from build123d import *

# Parameters (mm, degrees)
F1_W         = 18.1
F1_H         = 18.1
F2_DEPTH     = 5
F3_W         = 16.1
F3_H         = 16.1
F4_DEPTH     = 4
F5_ANGLE     = 45
F7_DEPTH     = 5
F9_DEPTH     = 8
F10_T1_DEPTH = 17.995241473
F11_T1_DEPTH = 15.801577482
F11_T3_DEPTH = 15.801577482
F11_T6_ANGLE = 128.9448568851
F11_T8_ANGLE = 128.9448568851


# Not quite as in the source:
# - a fillet or chamfer that OpenCascade refuses, or shapes differently, is made with other operations: its cross-section is extruded or revolved along the edge and cut away or added


with BuildPart() as f2:
    # F1 (on Top) → F2 (new body)
    with BuildSketch(Plane.XY):
        Rectangle(F1_W, F1_H)
    extrude(amount=F2_DEPTH)

    # F3 (on Top) → F4 (cut)
    with BuildSketch(Plane.XY):
        Rectangle(F3_W, F3_H)
    extrude(amount=F4_DEPTH, mode=Mode.SUBTRACT)


with BuildPart() as f2_1:
    # F5: moved
    add(f2.part.rotate(Axis((0, 0, 23.8891355693), (0, 0, 1)), F5_ANGLE))

    # F6 (on face) → F7 (join)
    with BuildSketch(Plane.XY.offset(5)):
        Polygon((12.7986327395, 0), (6.3993163697, -6.3993163697), (16.6505072266, 0), (6.3993163697, 6.3993163697), align=None)
    extrude(amount=-F7_DEPTH)

    # F8 (on face) → F9 (join)
    with BuildSketch(Plane(origin=(0, 0, 0), x_dir=(1, 0, 0), z_dir=(0, 0, -1))):
        Polygon((16.6505072266, 0), (6.3993163697, 6.3993163697), (6.3993163697, 4.9851028074), (11.3844191771, 0), (6.3993163697, -4.9851028074), (6.3993163697, -6.3993163697), align=None)
    extrude(amount=F9_DEPTH)

    # F10: fillet of radius 5 on 2 edges, made by hand

    # F10_s2 → F10_t1 (cut)
    with BuildSketch(Plane.XY.offset(-17.995241473)):
        with BuildLine():
            ThreePointArc((6.3993163697, -4.9851028074), (8.1578886795, -4.9366807501), (9.7908366557, -4.2821563649))
            Line((9.7908366557, -4.2821563649), (6.3993163697, -6.3993163697))
            Line((6.3993163697, -6.3993163697), (6.3993163697, -4.9851028074))
        make_face()
        with BuildLine():
            ThreePointArc((9.7908366557, 4.2821563649), (8.1578886795, 4.9366807501), (6.3993163697, 4.9851028074))
            Line((6.3993163697, 4.9851028074), (6.3993163697, 6.3993163697))
            Line((6.3993163697, 6.3993163697), (9.7908366557, 4.2821563649))
        make_face()
    extrude(amount=F10_T1_DEPTH, mode=Mode.SUBTRACT)

    # F11: chamfer of 3 on 2 edges, made by hand

    # F11_s2 → F11_t1 (cut)
    with BuildSketch(Plane(origin=(5.1217894323, -3.1972822879, 0), x_dir=(0, 0, 1), z_dir=(0.8482837296, -0.5295419852, 0))):
        Polygon((-5, -8.8171426514), (-8, -5.8171426514), (-8, -8.8171426514), align=None)
    extrude(amount=F11_T1_DEPTH, mode=Mode.SUBTRACT)

    # F11_s4 → F11_t3 (cut)
    with BuildSketch(Plane(origin=(18.5260105123, 11.564880997, 0), x_dir=(0, 0, 1), z_dir=(-0.8482837296, -0.5295419852, 0))):
        Polygon((-5, -8.8171426514), (-8, -5.8171426514), (-8, -8.8171426514), align=None)
    extrude(amount=F11_T3_DEPTH, mode=Mode.SUBTRACT)

    # F11_s5 → F11_t6 (revolve, cut)
    with BuildSketch(Plane(origin=(5.1217894331, 3.1972822878, 0), x_dir=(0, 0, 1), z_dir=(0.8482837296, 0.5295419851, 0))):
        Polygon((-8, 5.8171426509), (-5, 8.8171426509), (-8, 8.8171426509), align=None)
    revolve(axis=Axis((7.1431267295, -0.0407377158, -8), (0, 0, -1)), revolution_arc=F11_T6_ANGLE, mode=Mode.SUBTRACT)

    # F11_s7 → F11_t8 (revolve, cut)
    with BuildSketch(Plane(origin=(0.1002908696, -0.8203136168, 0), x_dir=(0, 0, 1), z_dir=(0.1213555739, -0.9926090996, 0))):
        Polygon((-8, -5.0952763393), (-5, -2.0952763393), (-8, -2.0952763393), align=None)
    revolve(axis=Axis((7.1431267295, 0.0407377158, -8), (0, 0, -1)), revolution_arc=F11_T8_ANGLE, mode=Mode.SUBTRACT)


solid = f2_1.part
The model under review builds one solid part; all positions refer to its coordinate system, in mm. A direction names the side the tool comes from. Round coordinates to 2 decimals unless told otherwise and drop trailing zeros. Write each loop counter-clockwise with the first axis right and the second up, starting at its lowest first coordinate (ties: lowest second). Pieces come first, ordered by that corner, then holes. Notation, with made-up numbers: (82, 82.5) -> (121, 82.5) arc R22 ccw to (121, 111.5) -> close; hole circle Ø8 at (79, 12.5). An arc over 180 degrees is marked (long way). Answer as a JSON object with one key per item and string values.
1. We need section B-B on y = -9.25. State the section outline as (x, z) points, and give its area (3 significant figures).
Results found:
{"outline": "(-3.55, 0) -> (-2.13, 0) -> (-2.13, 4) -> (2.13, 4) -> (2.13, 0) -> (3.55, 0) -> (3.55, 5) -> (-3.55, 5) -> close", "area": "18.4 mm^2"}
2. We need section C-C on x = 3.75. State the section outline as (y, z) points.
Results found:
{"outline": "(-9.05, 0) -> (-7.63, 0) -> (-7.63, 4) -> (7.63, 4) -> (7.63, 0) -> (9.05, 0) -> (9.05, 5) -> (-9.05, 5) -> close"}
3. The part is to be moulded in two halves that separate along Y. For faces 4 (the face through (2, 0, 5)), 5 (the face through (-5.772, 5.613, 1.972)), 6 (the face through (3.2, -9.6, 2.5)), 7 (the face through (6.877, -4.507, -0.502)), say which applies: pulls with the +Y half, pulls with the -Y half, needs draft (parallel to the pull), parting line crosses it, or undercut.
Results found:
{"face 4": "needs draft", "face 5": "undercut", "face 6": "pulls with the -Y half", "face 7": "undercut"}
4. Machinability: for faces 1 (the face through (7.037, 4.348, -0.502)), 2 (the face through (8.182, 4.932, -2.535)), 3 (the face through (8.134, -4.942, -2.535)), which of the approach directions +Z, -Z, +X, -X, +Y, -Y give a long, thin tool a straight path to every point of the face, cutting with its end or side? Answer none if there is none.
Results found:
{"face 1": "-Z", "face 2": "-Z, +Y", "face 3": "-Z, -Y"}
5. To check wall thickness, follow line 1 along X through (y, z) = (10.5, 0.75); line 2 along Y through (x, z) = (6, 1); line 3 along Z through (x, y) = (-1.5, 5.25). State the ranges of each line that lie inside material, in increasing order.
Results found:
{"line 1": "x = -2.3 to -0.88, 0.88 to 2.3", "line 2": "y = -6.8 to -5.38, 5.38 to 6.8", "line 3": "z = 4 to 5"}
6. We need section D-D on z = -0.5. State the section outline as (x, y) points, and give its area (3 significant figures).
Results found:
{"outline": "(6.4, -4.99) arc R5 ccw to (9.79, -4.28) -> (16.65, 0) -> (9.79, 4.28) arc R5 ccw to (6.4, 4.99) -> (11.38, 0) -> close", "area": "37.4 mm^2"}
7. Clearance check with flat-ended pins moving along their axes: pin 1 (1.5 mm diameter, centred on x = 0, y = 0.5, fed in from -Z); pin 2 (1.5 mm diameter, centred on y = -5.5, z = 2, fed in from -X). State where each tip first meets the part, or that it passes through.
Results found:
{"pin 1": "stops at z = 4", "pin 2": "stops at x = -8.05"}
8. We need section A-A on z = 3.5. State the section outline as (x, y) points, and give its area (3 significant figures).
Results found:
{"outline": "(-12.8, 0) -> (0, -12.8) -> (6.4, -6.4) -> (16.65, 0) -> (6.4, 6.4) -> (0, 12.8) -> close; hole (-11.38, 0) -> (0, -11.38) -> (11.38, 0) -> (0, 11.38) -> close", "area": "93.0 mm^2"}
